```python
from build123d import *

# Parameters (mm, degrees)
BOSS_EXTRUDE1_DEPTH                               = 6.35
BOSS_EXTRUDE2_DEPTH                               = 10.16
BOSS_EXTRUDE3_DEPTH                               = 3.81
F_5_1_5_1_DIAMETER_HOLE1_D                        = 5.1
F_5_1_5_1_DIAMETER_HOLE1_DEPTH                    = 8.128
F_5_1_5_1_DIAMETER_HOLE1_TIP                      = 1.532194579
CSK_FOR_6_FLAT_HEAD_MACHINE_SCREW_100_D           = 3.7973
CSK_FOR_6_FLAT_HEAD_MACHINE_SCREW_100_CSINK_D     = 7.0866
CSK_FOR_6_FLAT_HEAD_MACHINE_SCREW_100_CSINK_ANGLE = 100
FILLET1_R                                         = 5.08
FILLET2_R                                         = 2.54


with BuildPart() as part:
    # Sketch2 → Boss-Extrude1 (new body)
    with BuildSketch(Plane.XY):
        Polygon((30.619607592, -39.675283942), (66.760752948, -60.541383942), (85.810752948, -27.545816058), (49.669607592, -6.679716058), align=None)
    extrude(amount=BOSS_EXTRUDE1_DEPTH)

    # Sketch3 → Boss-Extrude2 (add)
    with BuildSketch(Plane.XY.offset(6.35)):
        Polygon((80.311491634, -24.370816058), (61.261491634, -57.366383942), (66.760752948, -60.541383942), (85.810752948, -27.545816058), align=None)
    extrude(amount=BOSS_EXTRUDE2_DEPTH)

    # Sketch4 → Boss-Extrude3 (add)
    with BuildSketch(Plane(origin=(9.525, 16.497783942, 0), x_dir=(0.8660254037844388, -0.4999999999999997, 0), z_dir=(0.49999999999999983, 0.8660254037844389, 0))):
        Polygon((46.355, -6.35), (81.7372, -16.51), (81.7372, -6.35), align=None)
    boss_extrude3 = extrude(amount=-BOSS_EXTRUDE3_DEPTH)

    # Mirror1: Boss-Extrude3 across plane
    add(boss_extrude3.mirror(Plane(origin=(0, 0, 0), x_dir=(0, 0, 1), z_dir=(0.4999999999999997, 0.8660254037844389, 0))))

    # Ø5.1 (5.1) Diameter Hole1
    with Locations(Plane(origin=(76.285752948, -44.0436, 0), x_dir=(0, 0, -1), z_dir=(0.8660254037844385, -0.5000000000000004, 0))):
        with Locations((-6.937306149, 9.733087598), (-6.937306149, -9.733087598)):
            Hole(F_5_1_5_1_DIAMETER_HOLE1_D / 2, depth=F_5_1_5_1_DIAMETER_HOLE1_DEPTH)
            with Locations((0, 0, -(F_5_1_5_1_DIAMETER_HOLE1_DEPTH + F_5_1_5_1_DIAMETER_HOLE1_TIP / 2))):  # 118° drill point
                Cone(0, F_5_1_5_1_DIAMETER_HOLE1_D / 2, F_5_1_5_1_DIAMETER_HOLE1_TIP, mode=Mode.SUBTRACT)

    # CSK for #6 Flat Head Machine Screw (100)1 (through all)
    with Locations(Plane.XY.offset(6.35)):
        with Locations((40.881368906, -34.601391971), (50.406368906, -18.103608029), (64.704448323, -26.358608029), (55.179448323, -42.856391971)):
            CounterSinkHole(CSK_FOR_6_FLAT_HEAD_MACHINE_SCREW_100_D / 2, CSK_FOR_6_FLAT_HEAD_MACHINE_SCREW_100_CSINK_D / 2, counter_sink_angle=CSK_FOR_6_FLAT_HEAD_MACHINE_SCREW_100_CSINK_ANGLE)

    # Fillet1
    # the kernel refuses this fillet: 5.08 mm, written as the material it takes off along each edge
    with BuildSketch(Plane(origin=(49.669607592, -6.679716058, -12.7), x_dir=(0.8660254037844385, -0.5000000000000002, 0), z_dir=(0, 0, 1))) as fillet1_piece_1:
        with BuildLine():
            CenterArc((FILLET1_R, -FILLET1_R), FILLET1_R, 90, 90)
            Line((0, -FILLET1_R), (0, 0))
            Line((0, 0), (FILLET1_R, 0))
        make_face()
    extrude(amount=31.75, mode=Mode.SUBTRACT)
    with BuildSketch(Plane(origin=(30.619607592, -39.675283942, -12.7), x_dir=(0.8660254037844386, -0.5, 0), z_dir=(0, 0, 1))) as fillet1_piece_2:
        with BuildLine():
            CenterArc((FILLET1_R, FILLET1_R), FILLET1_R, 180, 90)
            Line((0, FILLET1_R), (0, 0))
            Line((0, 0), (FILLET1_R, 0))
        make_face()
    extrude(amount=31.75, mode=Mode.SUBTRACT)

    # Fillet2
    fillet2_edges = [part.edges().sort_by_distance(p)[0] for p in [
        (85.810752948, -27.545816058, 8.255),
        (66.760752948, -60.541383942, 8.255),
    ]]
    fillet(fillet2_edges, radius=FILLET2_R)


solid = part.part
```
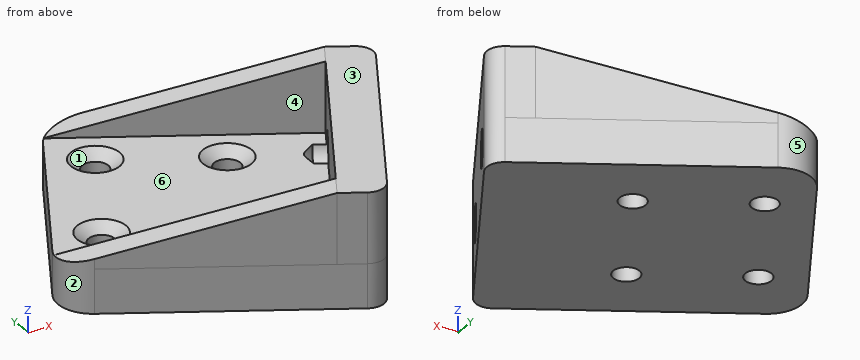
The listing builds one solid part. Answer for the finished solid, in the listing's coordinates (mm). Face numbers are marked on the shaded views. A direction names the side the tool comes from. Give positions to 0.01 mm unless a question says otherwise; leave off trailing zeros. Order: outer loops, then holes, each group sorted by start corner. A loop starts at its lowest first (then second) coordinate and runs counter-clockwise, first axis right, second up. Notation, with made-up numbers: (-18.5, -7) -> (25.5, -7) arc R13 ccw to (25.5, 5) -> close; hole circle Ø2 at (9.5, -27.75). An arc over 180 degrees is marked (long way). Write each question's results on one line, items separated by ' | '.
Q1. The part is cut by section D-D, the plane z = 11. Give the vertices of the cut face in (x, y).
Checked values:
outline: (44.64, -47.77) -> (64.56, -59.27) arc R2.54 ccw to (68.03, -58.34) -> (84.54, -29.75) arc R2.54 ccw to (83.61, -26.28) -> (63.69, -14.78) -> (61.79, -18.08) -> (78.41, -27.67) -> (63.17, -54.07) -> (46.55, -44.47) -> close
Q2. Which of the six approach directions +Z, -Z, +X, -X, +Y, -Y give full straight-line access (tool end or side, diameter ignored) to the marked faces 4, 5 and 6?
Checked values:
face 4: +Z, -X | face 5: +Z, -Z, +Y | face 6: +Z
Q3. The part is cut by section C-C, the plane y = -12. Give the vertices of the cut face in (x, z).
Checked values:
outline: (46.6, 0) -> (58.88, 0) -> (58.88, 9.41) -> (51.26, 7.51) -> (51.26, 6.35) -> (46.6, 6.35) -> close
Q4. The part is cut by section B-B, the plane z = 2.75. Give the vertices of the cut face in (x, y), and give its area (3 significant figures).
Checked values:
outline: (33.16, -35.28) arc R5.08 ccw to (35.02, -42.22) -> (64.56, -59.27) arc R2.54 ccw to (68.03, -58.34) -> (84.54, -29.75) arc R2.54 ccw to (83.61, -26.28) -> (54.07, -9.22) arc R5.08 ccw to (47.13, -11.08) -> close; hole circle Ø3.8 at (40.88, -34.6); hole circle Ø3.8 at (50.41, -18.1); hole circle Ø3.8 at (55.18, -42.86); hole circle Ø3.8 at (64.7, -26.36) | area: 1,530 mm^2
Q5. Straight lines are drawn through the part: probe 1 along Z at (x, y) = (65, -38); probe 2 along Y at (x, z) = (68.5, 11.75). For each, find the intervals that lie inside material, in ascending order. Write a range as from..to.
Checked values:
probe 1: z = 0..6.35 | probe 2: y = -57.53..-44.83, -21.95..-17.55
Q6. The part is cut by section A-A, the plane z = 14. Give the vertices of the cut face in (x, y).
Checked values:
outline: (53.69, -53) -> (64.56, -59.27) arc R2.54 ccw to (68.03, -58.34) -> (84.54, -29.75) arc R2.54 ccw to (83.61, -26.28) -> (72.74, -20) -> (70.84, -23.3) -> (78.41, -27.67) -> (63.17, -54.07) -> (55.6, -49.7) -> close
Q7. Determine the mould class of the marked faces 1, 2 and 3 for opening direction X: pulls with the +X half, pulls with the -X half, needs draft (parallel to the pull), parting line crosses it, or undercut.
Checked values:
face 1: undercut | face 2: pulls with the -X half | face 3: needs draft
Q8. Each of these flat-tipped pins is pushed along its axis until it touches: P1, Ø1.5, axis at x = 76.5, z = 9.5, coming from the -Y side; P2, Ø3, axis at x = 77.5, z = 11.5, coming from the -Y side; P3, Ø5, axis at x = 69, z = 13, coming from the -Y side; P4, Ø3.5, axis at x = 64.7, y = -26.36, coming from the +Z side. Where does it stop, or does it pass through?
Checked values:
P1: stops at y = -44.97 | P2: stops at y = -44.54 | P3: stops at y = -59.52 | P4: passes through
